Geometry: final body of the model. Coordinates: model frame, mm. A direction names the side the tool comes from. Coordinates: 2 decimals unless noted, no trailing zeros. Loops run counter-clockwise (first coordinate to the right, second up) from the corner with the lowest first, then second, coordinate; pieces in that order, holes last. Notation, with made-up numbers: M 65,26.25 L 89,26.25 A19 ccw 89,51.25 Z; hole C 31.5,42.25 d8. An arc over 180 degrees is marked long. Write each question's results on one line, items separated by ' | '. Start each with the question number.
from build123d import *

# Parameters (mm, degrees)
SKETCH2_R          = 2.5
CUT_EXTRUDE1_DEPTH = 100.36297097


with BuildPart() as part:
    # Sketch1 → Revolve1 (revolve)
    with BuildSketch(Plane.XY, mode=Mode.PRIVATE) as revolve1_sk:
        Polygon((5, 12), (34, 12), (34, 16), (28, 16), (28, 42), (9, 48), (9, 68), (0, 68), (0, 64), (5, 64), (5, 40), (20, 40), (20, 16), (5, 16), align=None)
    revolve(revolve1_sk.sketch.rotate(Axis((0, 0, 0), (1, 0, 0)), 90), axis=Axis((0, 0, 0), (1, 0, 0)))

    # Sketch2 → Cut-Extrude1 (cut, through all)
    with BuildSketch(Plane(origin=(9, 0, 0), x_dir=(0, 0, -1), z_dir=(1, 0, 0))):
        with Locations((0, 56)):
            Circle(SKETCH2_R)
        with Locations((39.597979746, 39.597979746)):
            Circle(SKETCH2_R)
        with Locations((56, 0)):
            Circle(SKETCH2_R)
        with Locations((39.597979746, -39.597979746)):
            Circle(SKETCH2_R)
        with Locations((0, -56)):
            Circle(SKETCH2_R)
        with Locations((-39.597979746, -39.597979746)):
            Circle(SKETCH2_R)
        with Locations((-56, 0)):
            Circle(SKETCH2_R)
        with Locations((-39.597979746, 39.597979746)):
            Circle(SKETCH2_R)
    extrude(amount=-CUT_EXTRUDE1_DEPTH, mode=Mode.SUBTRACT)


solid = part.part
Item 1: Pull-direction query (Y, two-part tool) for faces 1 (the cylindrical face through (30.96, 15.62, -3.47)), 2 (the flat face through (28, -1, -18)), 3 (the cylindrical face through (7.03, -37.49, -40.94)); classes: released by +Y, released by -Y, zero draft, split by the parting line, or undercut.
Item 2: Set-up query: faces 4 (the cylindrical face through (7.03, 53.56, 0.54)), 5 (the cylindrical face through (12.4, 15.62, -3.47)). Return all of +Z, -Z, +X, -X, +Y, -Y with unobstructed straight access to the full face (end or side cutting, diameter ignored); none if empty.
Item 3: Section A-A, the plane z = -56. Return loops of the section in (x, y).
Item 4: Section C-C, the plane y = 0. Count the separate pieces of the cut face and the enclosed holes in it, plus the area to 3 significant figures.
Item 5: Ray query, L1, parallel to Y at x = 6.9, z = 0; L2, parallel to X at y = -20, z = 57.5; L3, parallel to Z at x = 15, y = 10. Return the intervals inside material, ascending. Write a range as [from, to].
Item 6: Contact query for flat-ended pins moving along their axis: P1, Ø4, axis at y = 11, z = 48, coming from the -X side; P2, Ø4, axis at y = -39.6, z = -39.6, coming from the +X side; P3, Ø1.5, axis at x = 12.5, z = 23.5, coming from the +Y side; P4, Ø3, axis at x = 28, z = 29.5, coming from the -Y side. Output: stop coordinate, or through.
Solutions:
1) face 1: split by the parting line | face 2: zero draft | face 3: undercut
2) face 4: +X, -X | face 5: -X
3) outline: M 0,-38.57 L 9,-38.57 L 9,-2.5 L 5,-2.5 L 5,-30.98 L 0,-30.98 Z; M 0,30.98 L 5,30.98 L 5,2.5 L 9,2.5 L 9,38.57 L 0,38.57 Z
4) separate pieces: 4 | enclosed holes: 0 | area: 1,030 mm²
5) L1: y = [-68, -58.5], [-53.5, -40], [-16, -12], [12, 16], [40, 53.5], [58.5, 68] | L2: x = [5, 9] | L3: z = [-45.01, -38.73], [-12.49, -6.63], [6.63, 12.49], [38.73, 45.01]
6) P1: stops at x = 5 | P2: passes through | P3: stops at y = 41.09 | P4: stops at y = -31.45
